from build123d import *

# Parameters (mm, degrees)
BOSS_EXTRUDE1_DEPTH = 419.1
BOSS_EXTRUDE2_DEPTH = 0.0254


with BuildPart() as part:
    # Sketch1 → Boss-Extrude1 (new body)
    with BuildSketch(Plane(origin=(0, 0, 0), x_dir=(0, 0, -1), z_dir=(1, 0, 0))):
        with BuildLine():
            Line((0, 0), (57.15, 0))
            ThreePointArc((57.15, 0), (79.600640303, 9.299359697), (88.9, 31.75))
            Line((88.9, 31.75), (88.9, 95.25))
            ThreePointArc((88.9, 95.25), (79.600640303, 117.700640303), (57.15, 127))
            Line((57.15, 127), (0, 127))
            Line((0, 127), (0, 0))
        make_face()
    extrude(amount=BOSS_EXTRUDE1_DEPTH)

    # Sketch2 → Boss-Extrude2 (add)
    # profile 1 of 4: a face of its own
    with BuildSketch(Plane(origin=(0, 0, -88.9), x_dir=(-1, 0, 0), z_dir=(0, 0, -1))):
        Polygon((-259.290402428, 87.225987453), (-258.364360761, 87.225987453), (-258.364360761, 52.056756684), (-252.5028223, 52.056756684), (-252.5028223, 46.846500274), (-258.364360761, 46.846500274), (-258.364360761, 35.123423351), (-262.92333512, 35.123423351), (-262.92333512, 46.846500274), (-287.020771018, 46.846500274), align=None)
        Polygon((-262.92333512, 52.056756684), (-262.92333512, 74.118936171), (-278.065642812, 52.056756684), align=None, mode=Mode.SUBTRACT)
    # profile 2 of 4: a face of its own
    with BuildSketch(Plane(origin=(0, 0, -88.9), x_dir=(-1, 0, 0), z_dir=(0, 0, -1))):
        Polygon((-237.146812684, 85.923423351), (-227.754104351, 85.923423351), (-227.754104351, 35.123423351), (-232.31307871, 35.123423351), (-232.31307871, 80.71316694), (-240.128463325, 80.71316694), align=None)
    # profile 3 of 4: a face of its own
    with BuildSketch(Plane(origin=(0, 0, -88.9), x_dir=(-1, 0, 0), z_dir=(0, 0, -1))):
        Polygon((-181.136556274, 87.225987453), (-180.210514607, 87.225987453), (-180.210514607, 52.056756684), (-174.348976146, 52.056756684), (-174.348976146, 46.846500274), (-180.210514607, 46.846500274), (-180.210514607, 35.123423351), (-184.769488966, 35.123423351), (-184.769488966, 46.846500274), (-208.866924864, 46.846500274), align=None)
        Polygon((-184.769488966, 52.056756684), (-184.769488966, 74.118936171), (-199.911796659, 52.056756684), align=None, mode=Mode.SUBTRACT)
    # profile 4 of 4: a face of its own
    with BuildSketch(Plane(origin=(0, 0, -88.9), x_dir=(-1, 0, 0), z_dir=(0, 0, -1))):
        with BuildLine():
            Line((-146.343847941, 87.225987453), (-142.833030633, 84.468215017))
            Line((-142.833030633, 84.468215017), (-156.255546659, 63.94265412))
            add(Edge.make_bspline(
                [(-156.255546659, 63.94265412), (-155.361898067, 64.085095297), (-153.618735447, 64.362942919), (-151.854293263, 64.408778242), (-150.994408838, 64.431115658)],
                knots=[0, 0, 0, 0, 1.025318673, 2, 2, 2, 2], degree=3))
            add(Edge.make_bspline(
                [(-150.994408838, 64.431115658), (-150.478099463, 64.41723838), (-149.461759822, 64.38992137), (-147.969592522, 64.179698623), (-146.53574168, 63.848408427), (-145.166150279, 63.365485398), (-143.855902428, 62.748594083), (-142.597479079, 62.009252766), (-141.414535618, 61.109284606), (-140.291838502, 60.103953247), (-139.272542346, 58.990461015), (-138.370101311, 57.808978757), (-137.612066734, 56.560737398), (-136.997039528, 55.246369173), (-136.519448719, 53.867900148), (-136.171285185, 52.427094009), (-135.965478524, 50.922957224), (-135.937531401, 49.900016851), (-135.92333512, 49.380394504)],
                knots=[0, 0, 0, 0, 1.04369286, 2.054478336, 3.041073146, 4.015093852, 4.984733326, 5.965804835, 6.960378782, 7.985147595, 9.009457201, 10.008161701, 10.986880575, 11.956520048, 12.937015923, 13.931873656, 14.949455224, 16, 16, 16, 16], degree=3))
            add(Edge.make_bspline(
                [(-135.92333512, 49.380394504), (-135.943990471, 48.669489087), (-135.984635313, 47.270595467), (-136.389638981, 45.233127843), (-137.018973254, 43.292095903), (-137.918532809, 41.478489873), (-139.03587711, 39.794795434), (-140.398443313, 38.302937822), (-141.9579088, 36.972412709), (-143.7212029, 35.859796636), (-145.618843636, 34.951158067), (-147.61240977, 34.298519696), (-149.682540922, 33.896713912), (-151.087590662, 33.846340593), (-151.79833512, 33.820859248)],
                knots=[0, 0, 0, 0, 1.031375318, 2.029502543, 3.004789286, 3.987476834, 4.960371455, 5.9300674, 6.912260825, 7.929083631, 8.949397511, 9.960523116, 10.96833055, 12, 12, 12, 12], degree=3))
            add(Edge.make_bspline(
                [(-151.79833512, 33.820859248), (-152.48191009, 33.843040063), (-153.83595242, 33.886976373), (-155.827788404, 34.2783677), (-157.741685913, 34.912745078), (-159.564235785, 35.78671232), (-161.252546395, 36.890638164), (-162.762984775, 38.219599244), (-164.088019675, 39.745188052), (-165.19073703, 41.467167949), (-166.065349482, 43.317593618), (-166.721248967, 45.247081488), (-167.104371583, 47.248601223), (-167.157908351, 48.605413186), (-167.184873582, 49.288807966)],
                knots=[0, 0, 0, 0, 1.012016664, 2.004627821, 2.994792927, 3.992885782, 4.990978636, 5.973936114, 6.964471063, 7.975201453, 8.993600317, 9.990122807, 10.98767138, 12, 12, 12, 12], degree=3))
            add(Edge.make_bspline(
                [(-167.184873582, 49.288807966), (-167.167725751, 49.811969345), (-167.132713158, 50.880164923), (-166.888243378, 52.497985671), (-166.495417214, 54.153355657), (-166.055485638, 55.557673667), (-165.590656784, 56.708098043), (-165.203814209, 57.635611564), (-164.722317353, 58.59008657), (-164.208897991, 59.604252486), (-163.617341151, 60.651972481), (-162.974131154, 61.750757169), (-162.261484792, 62.883131662), (-161.761900716, 63.651578839), (-161.506508197, 64.04441694)],
                knots=[0, 0, 0, 0, 1.173818275, 2.396712641, 3.66331629, 4.989737886, 5.693666774, 6.447286557, 7.243889047, 8.091586357, 8.998013824, 9.943181721, 10.948533338, 12, 12, 12, 12], degree=3))
            Line((-161.506508197, 64.04441694), (-146.343847941, 87.225987453))
        make_face()
        with BuildLine():
            add(Edge.make_bspline(
                [(-151.950979351, 59.220859248), (-152.33796279, 59.2095665), (-153.093853864, 59.187508482), (-154.202852912, 59.059416254), (-155.252428104, 58.818202388), (-156.256484787, 58.510988198), (-157.196251446, 58.088578074), (-158.078558036, 57.575471964), (-158.906816503, 56.971370292), (-159.672351483, 56.284831354), (-160.366419739, 55.533165047), (-160.964134437, 54.728064553), (-161.479716702, 53.888932691), (-161.898915673, 53.008758216), (-162.225343058, 52.087877593), (-162.461465099, 51.130526202), (-162.592873831, 50.130284273), (-162.614735706, 49.451995376), (-162.625899223, 49.105634889)],
                knots=[0, 0, 0, 0, 1.129588631, 2.206414736, 3.251139165, 4.268635594, 5.265702196, 6.250456724, 7.242448911, 8.251968645, 9.246821453, 10.222880186, 11.173611482, 12.116736599, 13.062300278, 14.020270554, 14.989073742, 16, 16, 16, 16], degree=3))
            add(Edge.make_bspline(
                [(-162.625899223, 49.105634889), (-162.616808033, 48.762372324), (-162.598981564, 48.089285536), (-162.437113607, 47.097391158), (-162.189861555, 46.142860487), (-161.822063809, 45.230614425), (-161.383342118, 44.346747866), (-160.804144842, 43.523275723), (-160.162369779, 42.71018442), (-159.395232687, 41.969934491), (-158.57193359, 41.281135489), (-157.692350423, 40.679079238), (-156.77562872, 40.164022778), (-155.809392079, 39.760364562), (-154.807349249, 39.429086341), (-153.761151493, 39.195965442), (-152.67007119, 39.064168093), (-151.930975632, 39.04227774), (-151.554104351, 39.031115658)],
                knots=[0, 0, 0, 0, 0.989467248, 1.94019797, 2.891935182, 3.827694429, 4.772920941, 5.730924762, 6.725747692, 7.756678648, 8.79901574, 9.819492441, 10.826891316, 11.826466727, 12.835195252, 13.867842842, 14.912794438, 16, 16, 16, 16], degree=3))
            add(Edge.make_bspline(
                [(-151.554104351, 39.031115658), (-151.177233687, 39.042278616), (-150.43813934, 39.064170685), (-149.34705026, 39.195955593), (-148.30088495, 39.429122483), (-147.298724196, 39.760233548), (-146.332922854, 40.164508796), (-145.417002896, 40.675874945), (-144.545737995, 41.284838026), (-143.721898436, 41.968757384), (-142.957954417, 42.714397635), (-142.300787055, 43.516017606), (-141.739327555, 44.353403287), (-141.283082783, 45.22713266), (-140.919336041, 46.143412081), (-140.670830174, 47.097243388), (-140.509296495, 48.089324222), (-140.491424093, 48.76238539), (-140.482309479, 49.105634889)],
                knots=[0, 0, 0, 0, 1.087397944, 2.132534446, 3.165364764, 4.174271784, 5.174024072, 6.181601208, 7.194203697, 8.236725232, 9.267838612, 10.269026844, 11.221737037, 12.171628256, 13.107553087, 14.05945871, 15.010357665, 16, 16, 16, 16], degree=3))
            add(Edge.make_bspline(
                [(-140.482309479, 49.105634889), (-140.490296589, 49.452447228), (-140.505972688, 50.13312706), (-140.683278456, 51.130078776), (-140.929184911, 52.092741769), (-141.300504328, 53.01506583), (-141.782909034, 53.893411288), (-142.370496771, 54.732215095), (-143.050238077, 55.537908136), (-143.835425223, 56.286305469), (-144.690174904, 56.970611629), (-145.598995401, 57.574689762), (-146.549796847, 58.084503709), (-147.541615212, 58.509875365), (-148.585814766, 58.816844875), (-149.665537403, 59.058554803), (-150.794592696, 59.18718066), (-151.560607469, 59.209490063), (-151.950979351, 59.220859248)],
                knots=[0, 0, 0, 0, 0.978206639, 1.919901502, 2.851605144, 3.780102724, 4.718870031, 5.675451981, 6.667674623, 7.690630536, 8.733308323, 9.756129687, 10.767539656, 11.776269907, 12.797430371, 13.836405707, 14.897401972, 16, 16, 16, 16], degree=3))
        make_face(mode=Mode.SUBTRACT)
    extrude(amount=BOSS_EXTRUDE2_DEPTH)


solid = part.part
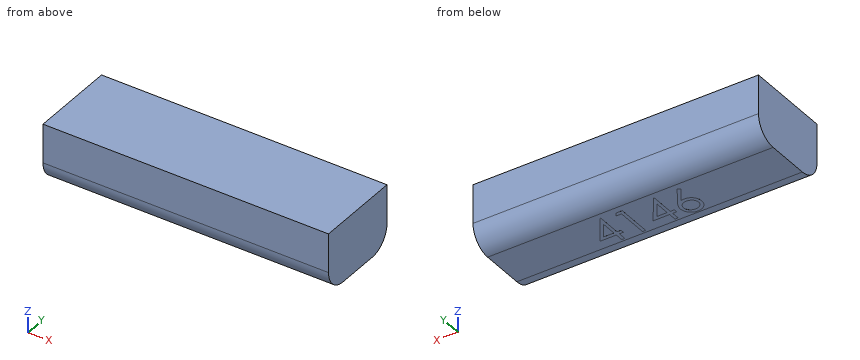
The model under review builds one solid part; all positions refer to its coordinate system, in mm. Round coordinates to 2 decimals unless told otherwise and drop trailing zeros. Order: outer loops, then holes, each group sorted by start corner. A loop starts at its lowest first (then second) coordinate and runs counter-clockwise, first axis right, second up. Notation, with made-up numbers: (-30, -20.5) -> (-3, -20.5) arc R15 ccw to (-3, -0.5) -> close; hole circle Ø11 at (-36.75, 55). An arc over 180 degrees is marked (long way). Write item = value, one per line. Start each with the question number.
Item 1: Consider section A-A on x = 121. Write out the cut boundary in (y, z).
Item 2: Clearance check with flat-ended pins moving along their axes: pin 1 Ø2 at (x, z) = (229.5, -64) entering from +Y; pin 2 Ø1.5 at (x, y) = (201, 108.5) entering from -Z; pin 3 Ø8 at (x, y) = (133.5, 78) entering from -Z. State where each tip first meets the part, or that it passes through.
Item 3: For line 1 along Z through (x, y) = (211, 66); line 2 along Y through (x, z) = (235.5, -74); line 3 along Z through (x, y) = (129, 116), list the stretches that pass through material, from the lowest coordinate up.
Item 4: Consider section B-B on y = 16. Write out the cut boundary in (x, z), plus the area to 3 significant figures.
Item 5: Consider section C-C on z = -82. Write out the cut boundary in (x, y).
Conclusion:
q1.outline = (0, -57.15) arc R31.75 ccw to (31.75, -88.9) -> (95.25, -88.9) arc R31.75 ccw to (127, -57.15) -> (127, 0) -> (0, 0) -> close
q2.pin_1 = 126.46
q2.pin_2 = -86.34
q2.pin_3 = -88.9
q3.line_1 = -88.9 to 0
q3.line_2 = 4.84 to 122.16
q3.line_3 = -81.18 to 0
q4.outline = (0, -84.72) -> (419.1, -84.72) -> (419.1, 0) -> (0, 0) -> close
q4.area = 35,500 mm2
q5.outline = (0, 11.99) -> (419.1, 11.99) -> (419.1, 115.01) -> (0, 115.01) -> close
